Can you work these out from the model? Positions are in its coordinate system, mm. A direction names the side the tool comes from. Coordinates: 2 decimals unless noted, no trailing zeros. Order: outer loops, then holes, each group sorted by start corner. A loop starts at its lowest first (then second) coordinate and runs counter-clockwise, first axis right, second up.
```python
from build123d import *

# Parameters (mm, degrees)
SKETCH1_W           = 7.62
SKETCH1_H           = 76.2
BOSS_EXTRUDE1_DEPTH = 7.62
SKETCH3_W           = 7.62
SKETCH3_H           = 7.740164582
BOSS_EXTRUDE3_DEPTH = 30.48
BOSS_EXTRUDE4_DEPTH = 2.54


with BuildPart() as part:
    # Sketch1 → Boss-Extrude1 (new body)
    with BuildSketch(Plane.XY):
        with Locations((3.81, 38.1)):
            Rectangle(SKETCH1_W, SKETCH1_H)
    extrude(amount=BOSS_EXTRUDE1_DEPTH)

    # Sketch3 → Boss-Extrude3 (add)
    with BuildSketch(Plane(origin=(7.62, 0, 0), x_dir=(0, 0, -1), z_dir=(1, 0, 0))):
        with Locations((-3.81, 72.329917709)):
            Rectangle(SKETCH3_W, SKETCH3_H)
    extrude(amount=BOSS_EXTRUDE3_DEPTH)

    # Sketch6 → Boss-Extrude4 (add)
    with BuildSketch(Plane(origin=(0, 68.459835418, 0), x_dir=(-1, 0, 0), z_dir=(0, -1, 0))):
        Polygon((-38.1, -7.62), (-38.1, -17.78), (-30.382577063, -17.78), (-30.382577063, 10.150655404), (-38.1, 10.150655404), (-38.1, 0), align=None)
    extrude(amount=-BOSS_EXTRUDE4_DEPTH)


solid = part.part
```
1. Imagine slicing it at A-A on z = 4.25. Please give me the cut outline in (x, y), then the cut area to 3 significant figures.
Completed:
outline: (0, 0) - (7.62, 0) - (7.62, 68.46) - (38.1, 68.46) - (38.1, 76.2) - (0, 76.2) - close
area: 817 mm2
2. Imagine slicing it at D-D on x = 25.5. Please give me the cut outline in (y, z), then the cut area to 3 significant figures.
Completed:
outline: (68.46, 0) - (76.2, 0) - (76.2, 7.62) - (68.46, 7.62) - close
area: 59.0 mm2
3. On a 3-axis mill with a long thin cutter (end or side, diameter ignored), from which of +Z, -Z, +X, -X, +Y, -Y can I reach the whole of each face in a straight line? I mean faces 1 (the flat face through (30.383, 70, 13)), 2 (the flat face through (34, 71, -5)), 3 (the flat face through (34, 71, 13)), 4 (the flat face through (7.62, 34, 4)). Say none if no direction works.
Completed:
face 1: +Z, -X, +Y, -Y
face 2: -Z, +X, -X, +Y
face 3: +Z, +X, -X, +Y
face 4: +Z, -Z, +X, -Y
4. Imagine slicing it at C-C on y = 9.5. Please give me the cut outline in (x, z).
Completed:
outline: (0, 0) - (7.62, 0) - (7.62, 7.62) - (0, 7.62) - close
5. Imagine slicing it at B-B on x = 36. Please give me the cut outline in (y, z).
Completed:
outline: (68.46, -10.15) - (71, -10.15) - (71, 0) - (76.2, 0) - (76.2, 7.62) - (71, 7.62) - (71, 17.78) - (68.46, 17.78) - close
6. Please list where these lines run through material, in increasing order: probe 1 along Y at (x, z) = (8.5, 5.75); probe 2 along X at (y, z) = (17, 7.5).
Completed:
probe 1: y = 68.46 to 76.2
probe 2: x = 0 to 7.62
7. I'm going to push flat-ended pins straight in: pin 1 (8 mm diameter, centred on y = 7.5, z = 13.5, fed in from -X); pin 2 (8.5 mm diameter, centred on x = 27.5, z = 7.5, fed in from -Y); pin 3 (2.5 mm diameter, centred on x = 32.5, z = 11.5, fed in from +Y); pin 4 (8.5 mm diameter, centred on y = 50.5, z = 4.5, fed in from +X). Where does each tip first touch, or does it pass through?
Completed:
pin 1: passes through
pin 2: stops at y = 68.46
pin 3: stops at y = 71
pin 4: stops at x = 7.62
